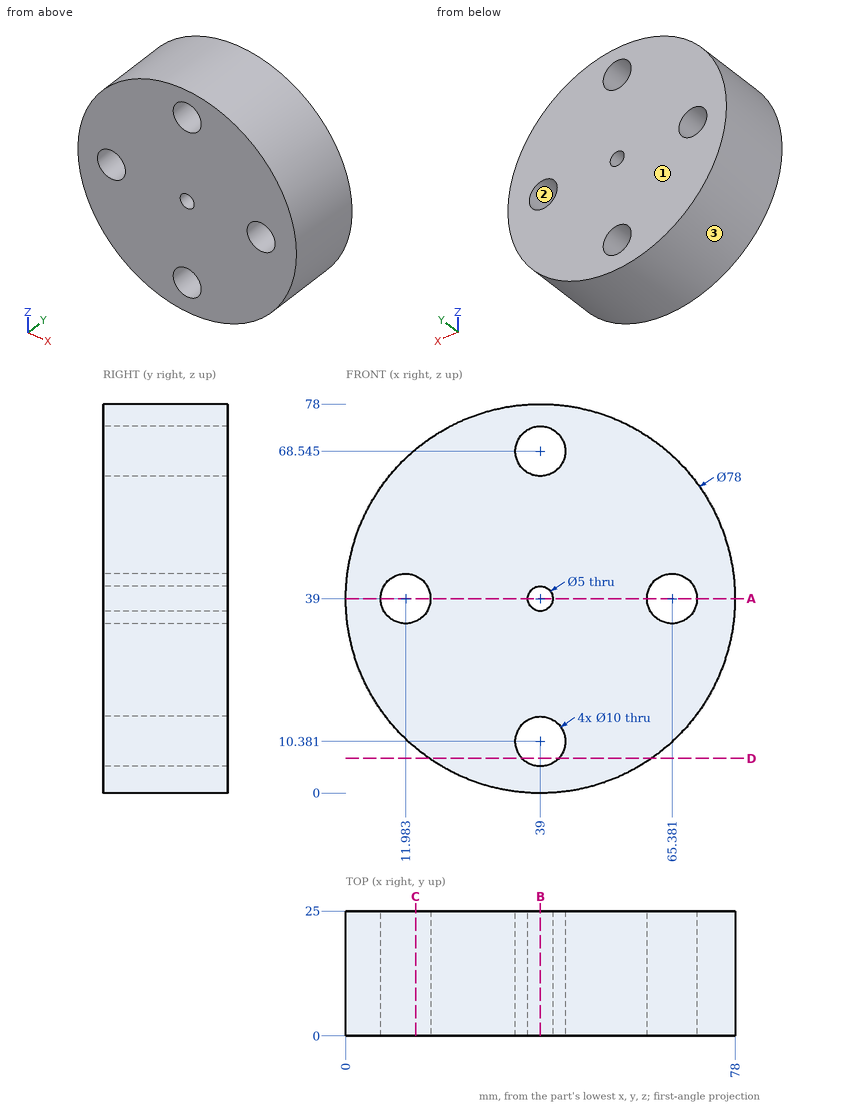
Part print with two shaded views. Sizes in mm from the minimum x, y, z corner. Coordinates: 2 decimals unless noted, no trailing zeros. Write each loop counter-clockwise with the first axis right and the second up, starting at its lowest first coordinate (ties: lowest second). Pieces come first, ordered by that corner, then holes.
(1) Mould opens along X. For the marked faces 1, 2 and 3 say: pulls with the +X half, pulls with the -X half, needs draft (parallel to the pull), parting line crosses it, or undercut.
(2) Cut at B-B on x = 39. List the corners of the cut face in (y, z) (1 decimal).
(3) Cut at C-C on x = 14. List the corners of the cut face in (y, z) (1 decimal).
(4) Cut at D-D on z = 7. List the corners of the cut face in (x, y).
(5) Drill centre lines: line 1 (Z direction, x = 39, y = 7) (1 decimal); line 2 (X direction, y = 9.5, z = 34.5) (1 decimal); line 3 (X direction, y = 15, z = 35) (1 decimal). Where is each one in solid material? Low to high.
(6) Pin check, flat tips, straight feed: pin 1 Ø4 at (y, z) = (3, 27.5) entering from +X (1 decimal); pin 2 Ø8 at (y, z) = (19.5, 15) entering from -X; pin 3 Ø4 at (x, y) = (40, 9.5) entering from +Z; pin 4 Ø8 at (x, z) = (39, 68.54) entering from -Y. Stop position of each tip, or through.
(7) Cut at A-A on z = 39. List the corners of the cut face in (x, y).
Working result:
1. face 1: needs draft
1. face 2: undercut
1. face 3: parting line crosses it
2. outline: (0, 0) - (25, 0) - (25, 5.4) - (0, 5.4) - close; (0, 15.4) - (25, 15.4) - (25, 36.5) - (0, 36.5) - close; (0, 41.5) - (25, 41.5) - (25, 63.5) - (0, 63.5) - close; (0, 73.5) - (25, 73.5) - (25, 78) - (0, 78) - close
3. outline: (0, 9.1) - (25, 9.1) - (25, 34.4) - (0, 34.4) - close; (0, 43.6) - (25, 43.6) - (25, 68.9) - (0, 68.9) - close
4. outline: (16.71, 0) - (35.32, 0) - (35.32, 25) - (16.71, 25) - close; (42.68, 0) - (61.29, 0) - (61.29, 25) - (42.68, 25) - close
5. line 1: z = 0 to 5.4, 15.4 to 36.5, 41.5 to 63.5, 73.5 to 78
5. line 2: x = 0.3 to 9.8, 14.2 to 63.2, 67.6 to 77.7
5. line 3: x = 0.2 to 9, 15 to 62.4, 68.4 to 77.8
6. pin 1: stops at x = 76.8
6. pin 2: stops at x = 5.52
6. pin 3: stops at z = 78
6. pin 4: passes through
7. outline: (0, 0) - (6.98, 0) - (6.98, 25) - (0, 25) - close; (16.98, 0) - (36.5, 0) - (36.5, 25) - (16.98, 25) - close; (41.5, 0) - (60.38, 0) - (60.38, 25) - (41.5, 25) - close; (70.38, 0) - (78, 0) - (78, 25) - (70.38, 25) - close
